from build123d import *

# Parameters (mm, degrees)
SKETCH_1_W          = 55
SKETCH_1_H          = 52
EXTRUDE_1_DEPTH     = 3
SKETCH_2_W          = 10
SKETCH_2_H          = 6
CUT_EXTRUDE_1_DEPTH = 38.963798545
SKETCH_3_R          = 1
CUT_EXTRUDE_2_DEPTH = 38.963798545
SKETCH_4_R          = 1.6
CUT_EXTRUDE_3_DEPTH = 38.963798545
CHAMFER_1_SIZE      = 0.5
SKETCH_5_W          = 8
SKETCH_5_H          = 15
CUT_EXTRUDE_4_DEPTH = 38.963798545
SKETCH_6_R          = 1
CUT_EXTRUDE_5_DEPTH = 38.963798545
SKETCH_7_R          = 2.1
CUT_EXTRUDE_6_DEPTH = 38.963798545
CHAMFER_2_SIZE      = 0.5
FILLET_1_R          = 2


with BuildPart() as part:
    # 草图1 → 凸台-拉伸1 (new body)
    with BuildSketch(Plane(origin=(0, 0, 0), x_dir=(1, 0, 0), z_dir=(0, 1, 0))):
        Rectangle(SKETCH_1_W, SKETCH_1_H)
    extrude(amount=EXTRUDE_1_DEPTH)

    # 草图2 → 切除-拉伸1 (cut, through all)
    with BuildSketch(Plane(origin=(0, 3, 0), x_dir=(1, 0, 0), z_dir=(0, 1, 0))):
        with Locations((0, -23)):
            Rectangle(SKETCH_2_W, SKETCH_2_H)
        with Locations((0, 23)):
            Rectangle(SKETCH_2_W, SKETCH_2_H)
    extrude(amount=-CUT_EXTRUDE_1_DEPTH, mode=Mode.SUBTRACT)

    # 草图3 → 切除-拉伸2 (cut, through all)
    with BuildSketch(Plane(origin=(0, 3, 0), x_dir=(1, 0, 0), z_dir=(0, 1, 0))):
        with Locations((-5, 20)):
            Circle(SKETCH_3_R)
        with Locations((5, 20)):
            Circle(SKETCH_3_R)
        with Locations((-5, -20)):
            Circle(SKETCH_3_R)
        with Locations((5, -20)):
            Circle(SKETCH_3_R)
    extrude(amount=-CUT_EXTRUDE_2_DEPTH, mode=Mode.SUBTRACT)

    # 草图4 → 切除-拉伸3 (cut, through all)
    with BuildSketch(Plane(origin=(0, 3, 0), x_dir=(1, 0, 0), z_dir=(0, 1, 0))):
        with Locations(Location((-11, -23, 0), (0, 0, 270))):
            Circle(SKETCH_4_R)
        with Locations(Location((11, -23, 0), (0, 0, 90))):
            Circle(SKETCH_4_R)
        with Locations(Location((11, 23, 0), (0, 0, 270))):
            Circle(SKETCH_4_R)
        with Locations(Location((-11, 23, 0), (0, 0, 90))):
            Circle(SKETCH_4_R)
    extrude(amount=-CUT_EXTRUDE_3_DEPTH, mode=Mode.SUBTRACT)

    # 倒角1
    chamfer_1_edges = [part.edges().sort_by_distance(p)[0] for p in [
        (5, 1.5, 26),
        (-5, 1.5, 26),
        (-5, 1.5, -26),
        (5, 1.5, -26),
    ]]
    chamfer(chamfer_1_edges, length=CHAMFER_1_SIZE)

    # 草图5 → 切除-拉伸4 (cut, through all)
    with BuildSketch(Plane(origin=(0, 3, 0), x_dir=(1, 0, 0), z_dir=(0, 1, 0))):
        with Locations((-23.5, 0)):
            Rectangle(SKETCH_5_W, SKETCH_5_H)
        with Locations((23.5, 0)):
            Rectangle(SKETCH_5_W, SKETCH_5_H)
    extrude(amount=-CUT_EXTRUDE_4_DEPTH, mode=Mode.SUBTRACT)

    # 草图6 → 切除-拉伸5 (cut, through all)
    with BuildSketch(Plane(origin=(0, 3, 0), x_dir=(1, 0, 0), z_dir=(0, 1, 0))):
        with Locations((19.5, 7.5)):
            Circle(SKETCH_6_R)
        with Locations((19.5, -7.5)):
            Circle(SKETCH_6_R)
        with Locations((-19.5, 7.5)):
            Circle(SKETCH_6_R)
        with Locations((-19.5, -7.5)):
            Circle(SKETCH_6_R)
    extrude(amount=-CUT_EXTRUDE_5_DEPTH, mode=Mode.SUBTRACT)

    # 草图7 → 切除-拉伸6 (cut, through all)
    with BuildSketch(Plane(origin=(0, 3, 0), x_dir=(1, 0, 0), z_dir=(0, 1, 0))):
        with Locations(Location((-23.5, 15, 0), (0, 0, 270))):
            Circle(SKETCH_7_R)
        with Locations(Location((-23.5, -15, 0), (0, 0, 90))):
            Circle(SKETCH_7_R)
        with Locations(Location((23.5, -15, 0), (0, 0, 270))):
            Circle(SKETCH_7_R)
        with Locations(Location((23.5, 15, 0), (0, 0, 90))):
            Circle(SKETCH_7_R)
    extrude(amount=-CUT_EXTRUDE_6_DEPTH, mode=Mode.SUBTRACT)

    # 倒角2
    chamfer_2_edges = [part.edges().sort_by_distance(p)[0] for p in [
        (-27.5, 1.5, 7.5),
        (-27.5, 1.5, -7.5),
        (27.5, 1.5, 7.5),
        (27.5, 1.5, -7.5),
    ]]
    chamfer(chamfer_2_edges, length=CHAMFER_2_SIZE)

    # 圆角1
    fillet_1_edges = [part.edges().sort_by_distance(p)[0] for p in [
        (27.5, 1.5, 26),
        (-27.5, 1.5, 26),
        (-27.5, 1.5, -26),
        (27.5, 1.5, -26),
    ]]
    fillet(fillet_1_edges, radius=FILLET_1_R)


solid = part.part
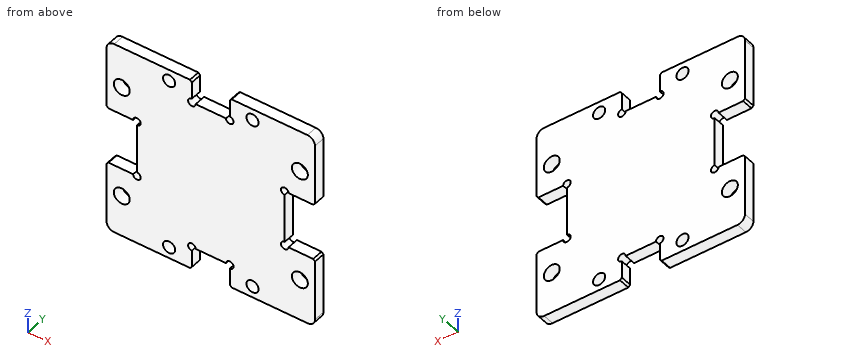
Input: part model. Units: mm. Frame: model coordinates. Coordinates: 2 decimals unless noted, no trailing zeros. Write each loop counter-clockwise with the first axis right and the second up, starting at its lowest first coordinate (ties: lowest second). Pieces come first, ordered by that corner, then holes. Notation, with made-up numbers: M 30.5,-38 L 50.5,-38 A22 ccw 50.5,-27 Z; hole C 61,8.5 d9. An arc over 180 degrees is marked long. Answer as a JSON object with one key per item and string values. Group by question number.
(1) Section D-D on y = 0.8. Give the number of separate pieces and of enclosed holes in the cut face, plus the area to 3 significant figures.
(2) Section C-C on z = 15. Output: boundary loops of the cut face in (x, y).
(3) Ray query, line 1 along X through (y, z) = (2.45, 23); line 2 along X through (y, z) = (0.85, -15); line 3 along Z through (x, y) = (19, 2.3). Return the intervals inside material, ascending. Write a range as [from, to].
(4) Section A-A on z = -23. Output: boundary loops of the cut face in (x, y).
(5) Contact query for flat-ended pins moving along their axis: P1, Ø1.8, axis at x = 19.5, z = -7.5, coming from the +Y side; P2, Ø1.5, axis at y = 2, z = 0.5, coming from the +X side. Output: stop coordinate, or through.
(6) Section B-B on x = 11. Output: boundary loops of the cut face in (y, z), plus the area to 3 significant figures.
Result set:
{
 "1": {"separate pieces": "1", "enclosed holes": "8", "area": "2,390 mm2"},
 "2": {"outline": "M -27.5,0 L -25.6,0 L -25.6,3 L -27.5,3 Z; M -21.4,0 L 21.4,0 L 21.4,3 L -21.4,3 Z; M 25.6,0 L 27.5,0 L 27.5,3 L 25.6,3 Z"},
 "3": {"line 1": "x = [-27.5, -12.6], [-9.4, -5], [5, 9.4], [12.6, 27.5]", "line 2": "x = [-27.5, -25.6], [-21.4, 21.4], [25.6, 27.5]", "line 3": "z = [-26, -8.37], [-6.63, 6.63], [8.37, 26]"},
 "4": {"outline": "M -27.5,0 L -12.6,0 L -12.6,3 L -27.5,3 Z; M -9.4,0 L -5,0 L -5,3 L -9.4,3 Z; M 5,0 L 9.4,0 L 9.4,3 L 5,3 Z; M 12.6,0 L 27.5,0 L 27.5,3 L 12.6,3 Z"},
 "5": {"P1": "passes through", "P2": "stops at x = 19.5"},
 "6": {"outline": "M 0,-26 L 3,-26 L 3,-24.6 L 0,-24.6 Z; M 0,-21.4 L 3,-21.4 L 3,21.4 L 0,21.4 Z; M 0,24.6 L 3,24.6 L 3,26 L 0,26 Z", "area": "137 mm2"}
}
